```python
from build123d import *

# Parameters (mm, degrees)
BOSS_EXTRUDE1_DEPTH = 32
SKETCH2_R           = 4
SKETCH2_R_2         = 1.85
CUT_EXTRUDE1_DEPTH  = 33
CIRPATTERN1_COUNT   = 2
CIRPATTERN1_ANGLE   = 90


with BuildPart() as part:
    # Sketch1 → Boss-Extrude1 (new body, symmetric)
    with BuildSketch(Plane.XY):
        with BuildLine():
            Line((-13.5, 16), (13.5, 16))
            ThreePointArc((13.5, 16), (15.267766953, 15.267766953), (16, 13.5))
            Line((16, 13.5), (16, -13.5))
            ThreePointArc((16, -13.5), (15.267766953, -15.267766953), (13.5, -16))
            Line((13.5, -16), (-13.5, -16))
            ThreePointArc((-13.5, -16), (-15.267766953, -15.267766953), (-16, -13.5))
            Line((-16, -13.5), (-16, 13.5))
            ThreePointArc((-16, 13.5), (-15.267766953, 15.267766953), (-13.5, 16))
        make_face()
        with BuildLine():
            Line((-13.5, 14), (13.5, 14))
            ThreePointArc((13.5, 14), (13.853553391, 13.853553391), (14, 13.5))
            Line((14, 13.5), (14, -13.5))
            ThreePointArc((14, -13.5), (13.853553391, -13.853553391), (13.5, -14))
            Line((13.5, -14), (-13.5, -14))
            ThreePointArc((-13.5, -14), (-13.853553391, -13.853553391), (-14, -13.5))
            Line((-14, -13.5), (-14, 13.5))
            ThreePointArc((-14, 13.5), (-13.853553391, 13.853553391), (-13.5, 14))
        make_face(mode=Mode.SUBTRACT)
    extrude(amount=BOSS_EXTRUDE1_DEPTH, both=True)

    # Sketch2 → Cut-Extrude1 (cut, through all)
    with BuildSketch(Plane(origin=(16, 0, 0), x_dir=(0, 0, -1), z_dir=(1, 0, 0))):
        Circle(SKETCH2_R)
        with Locations((16, 0)):
            Circle(SKETCH2_R)
        with Locations((32, 0)):
            Circle(SKETCH2_R)
        with Locations((-16, 0)):
            Circle(SKETCH2_R)
        with Locations((-32, 0)):
            Circle(SKETCH2_R)
        with Locations((24, 0)):
            Circle(SKETCH2_R_2)
        with Locations((16, 8)):
            Circle(SKETCH2_R_2)
        with Locations((16, -8)):
            Circle(SKETCH2_R_2)
        with Locations((8, 0)):
            Circle(SKETCH2_R_2)
        with Locations((-8, 0)):
            Circle(SKETCH2_R_2)
        with Locations((-24, 0)):
            Circle(SKETCH2_R_2)
        with Locations((-16, -8)):
            Circle(SKETCH2_R_2)
        with Locations((-16, 8)):
            Circle(SKETCH2_R_2)
        with Locations((0, 8)):
            Circle(SKETCH2_R_2)
        with Locations((0, -8)):
            Circle(SKETCH2_R_2)
    cut_extrude1 = extrude(amount=-CUT_EXTRUDE1_DEPTH, mode=Mode.SUBTRACT)

    # CirPattern1: Cut-Extrude1 ×2 about axis
    cirpattern1_axis = Axis((0, 0, -17.6), (0, 0, 1))
    for i in range(1, CIRPATTERN1_COUNT):
        add(cut_extrude1.rotate(cirpattern1_axis, i * CIRPATTERN1_ANGLE / (CIRPATTERN1_COUNT - 1)), mode=Mode.SUBTRACT)


solid = part.part
```
The model under review builds one solid part; all positions refer to its coordinate system, in mm. Round coordinates to 2 decimals unless told otherwise and drop trailing zeros. Order: outer loops, then holes, each group sorted by start corner. A loop starts at its lowest first (then second) coordinate and runs counter-clockwise, first axis right, second up. Notation, with made-up numbers: (63.25, 69.25) - (101.25, 69.25) arc R23 cw to (101.25, 91.25) - close; hole circle Ø9 at (-3.5, 10.5). An arc over 180 degrees is marked (long way). Answer in a Markdown table with one row per item.
(1) Take a section at B-B on y = 11.5. Write out the cut boundary in (x, z).
Result set:
| item | result |
|---|---|
| outline | (-16, -32) - (-14, -32) - (-14, 32) - (-16, 32) - close; (14, -32) - (16, -32) - (16, 32) - (14, 32) - close |
(2) For line 1 (Y direction, x = -10.5, z = -22); line 2 (Y direction, x = 15, z = 16), list the stretches that pass through material, from the lowest coordinate up. Write a range as from..to.
Result set:
| item | result |
|---|---|
| line 1 | y = -16..-14, 14..16 |
| line 2 | y = -15.5..-9.85, -6.15..-4, 4..6.15, 9.85..15.5 |
(3) Clearance check with a flat-ended pin moving along its axis: P1, Ø3.5, axis at x = -8, z = 16, coming from the -Y side. State where the tip first meets the part, or that it passes through.
Result set:
| item | result |
|---|---|
| P1 | passes through |
(4) Mouldability with a two-part tool opening along Z and no side actions: class faces 1 (the face through (-0.08, 15.01, 25.85)), 2 (the face through (-6, -14, 0)), 3 (the face through (-15, 0, 28)) as released by +Z, released by -Z, zero draft, split by the parting line, or undercut.
Result set:
| item | result |
|---|---|
| face 1 | undercut |
| face 2 | zero draft |
| face 3 | released by +Z |
(5) Take a section at A-A on z = -24. Count the separate pieces of the cut face and the enclosed holes in it, plus the area to 3 significant figures.
Result set:
| item | result |
|---|---|
| separate pieces | 4 |
| enclosed holes | 0 |
| area | 205 mm2 |
